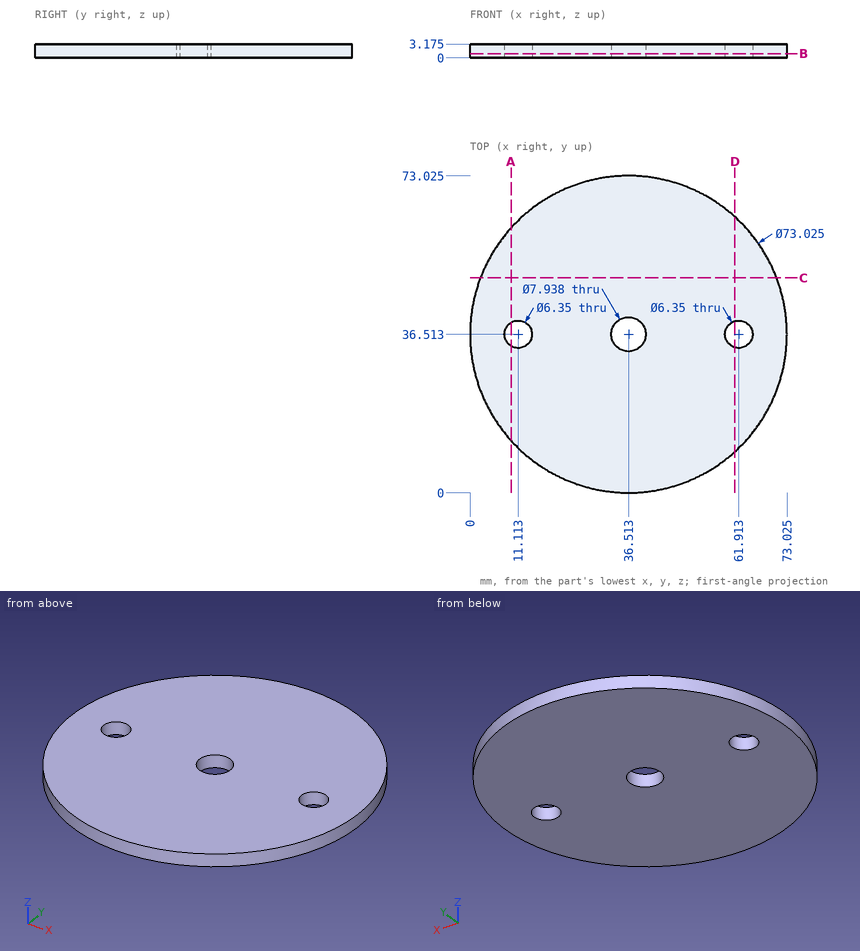
Part print with two shaded views. Sizes in mm from the minimum x, y, z corner. Coordinates: 2 decimals unless noted, no trailing zeros. Write each loop counter-clockwise with the first axis right and the second up, starting at its lowest first coordinate (ties: lowest second). Pieces come first, ordered by that corner, then holes. Notation, with made-up numbers: (-36.75, 27) - (-27.75, 27) arc R18 ccw to (-27.75, 34) - close; hole circle Ø8 at (-26, 59.25). An arc over 180 degrees is marked (long way). Use a Markdown table: item, result. Add a question column.
Item 1: Band-saw the part on B-B, the plane z = 0.95. Give the number of separate pieces and of enclosed holes in the cut face, and give its area (3 significant figures).
Item 2: Band-saw the part on A-A, the plane x = 9.5. Write the cut outline in (y, z) (1 decimal), and give its area (3 significant figures).
Item 3: Band-saw the part on D-D, the plane x = 61. Write the cut outline in (y, z) (1 decimal).
Item 4: Band-saw the part on C-C, the plane y = 49.5. Write the cut outline in (x, z) (1 decimal).
Item 5: Drop flat-ended pins along their axis: pin 1 (1.5 mm diameter, centred on y = 56, z = 1.5, fed in from -X) (1 decimal); pin 2 (1.5 mm diameter, centred on x = 65.5, z = 1, fed in from +Y); pin 3 (1 mm diameter, centred on x = 60, z = 2, fed in from +Y). Give the stop position or say it passes through.
Item 6: Drill centre lines: line 1 along X through (y, z) = (36.5, 0.25) (1 decimal); line 2 along X through (y, z) = (38, 0.5) (1 decimal); line 3 along Y through (x, z) = (30.5, 1). Where is each one in solid material? Low to high.
A:
| question | item | result |
|---|---|---|
| 1 | separate pieces | 1 |
| 1 | enclosed holes | 3 |
| 1 | area | 4,080 mm² |
| 2 | outline | (11.9, 0) - (33.8, 0) - (33.8, 3.2) - (11.9, 3.2) - close; (39.2, 0) - (61.1, 0) - (61.1, 3.2) - (39.2, 3.2) - close |
| 2 | area | 139 mm² |
| 3 | outline | (9.4, 0) - (33.5, 0) - (33.5, 3.2) - (9.4, 3.2) - close; (39.6, 0) - (63.6, 0) - (63.6, 3.2) - (39.6, 3.2) - close |
| 4 | outline | (2.4, 0) - (70.6, 0) - (70.6, 3.2) - (2.4, 3.2) - close |
| 5 | pin 1 | stops at x = 5.2 |
| 5 | pin 2 | stops at y = 59.66 |
| 5 | pin 3 | stops at y = 64.88 |
| 6 | line 1 | x = 0 to 7.9, 14.3 to 32.5, 40.5 to 58.7, 65.1 to 73 |
| 6 | line 2 | x = 0 to 8.3, 13.9 to 32.8, 40.2 to 59.1, 64.7 to 73 |
| 6 | line 3 | y = 0.5 to 72.53 |
